Geometry: final body of the model. Coordinates: model frame, mm. Face numbers are marked on the shaded views. A direction names the side the tool comes from. Coordinates: 2 decimals unless noted, no trailing zeros. Loops run counter-clockwise (first coordinate to the right, second up) from the corner with the lowest first, then second, coordinate; pieces in that order, holes last. Notation, with made-up numbers: (75.5, 4) - (92.5, 4) arc R27 cw to (92.5, 27) - close; hole circle Ø10 at (60.25, 49.5). An arc over 180 degrees is marked (long way). Return JSON: item names as keys, results as strings.
from build123d import *

# Parameters (mm, degrees)
F0_W      = 822.325
F0_H      = 177.8
F1_DEPTH  = 228.6
F2_T      = -19.05
F3_W      = 784.225
F3_H      = 209.55
F4_DEPTH  = 6.35
F5_W      = 158.75
F5_H      = 209.55
F6_DEPTH  = 6.35
F7_W      = 158.75
F7_H      = 209.55
F8_DEPTH  = 6.35
F9_W      = 784.225
F9_H      = 158.75
F10_DEPTH = 6.35


with BuildPart() as f1:
    # F0 (on Top) → F1 (new body)
    with BuildSketch(Plane.XY):
        Rectangle(F0_W, F0_H)
    extrude(amount=F1_DEPTH)

    # F2
    f2_openings = [f1.faces().sort_by_distance(p)[0] for p in [
        (0, 0, 0),
    ]]
    offset(amount=F2_T, openings=f2_openings)

    # F3 (on face) → F4 (cut)
    with BuildSketch(Plane.XZ.offset(88.9)):
        with Locations((0.143385, 104.775)):
            Rectangle(F3_W, F3_H)
    extrude(amount=-F4_DEPTH, mode=Mode.SUBTRACT)

    # F5 (on face) → F6 (cut)
    with BuildSketch(Plane(origin=(-411.1625, 0, 0), x_dir=(0, -1, 0), z_dir=(-1, 0, 0))):
        with Locations((-9.525, 104.775)):
            Rectangle(F5_W, F5_H)
    extrude(amount=-F6_DEPTH, mode=Mode.SUBTRACT)

    # F7 (on face) → F8 (cut)
    with BuildSketch(Plane.YZ.offset(411.1625)):
        with Locations((9.525, 104.775)):
            Rectangle(F7_W, F7_H)
    extrude(amount=-F8_DEPTH, mode=Mode.SUBTRACT)

    # F9 (on face) → F10 (cut)
    with BuildSketch(Plane.XY.offset(228.6)):
        with Locations((0, 9.525)):
            Rectangle(F9_W, F9_H)
    extrude(amount=-F10_DEPTH, mode=Mode.SUBTRACT)


solid = f1.part
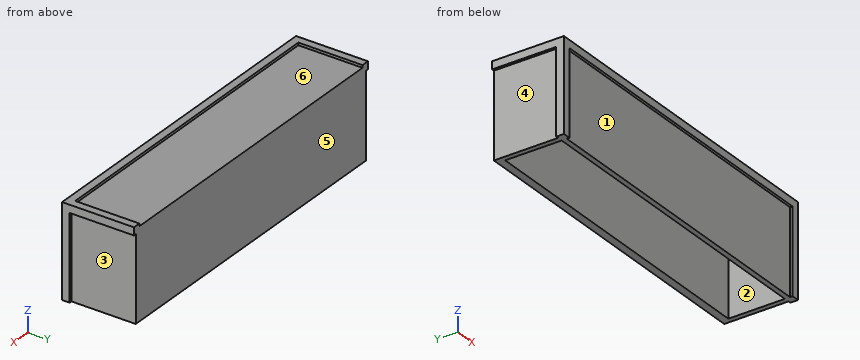
Item 1: First-contact query: pin 1 Ø3 at (y, z) = (50.5, 191.5) entering from -X; pin 2 Ø1.9 at (x, z) = (409, 112.5) entering from +Y; pin 3 Ø1.9 at (x, y) = (67, -87.5) entering from -Z. Flat tips, straight axial feed; report the tip coordinate or a pass-through.
Worked out:
{"pin 1": "x = -404.81", "pin 2": "y = -69.85", "pin 3": "z = 209.55"}
Item 2: Reachability of the marked faces 1, 2 and 3 from +Z, -Z, +X, -X, +Y, -Y: full face, straight path, thin tool, end or side. Return the list, or none.
Worked out:
{"face 1": "-Z, -Y", "face 2": "-Z", "face 3": "-Z, +X, +Y"}
Item 3: Ray query, probe 1 along X at (y, z) = (54, 103); probe 2 along Y at (x, z) = (-187, 156); probe 3 along Z at (x, y) = (194.5, 71). Return the intervals inside material, ascending. Write a range as from..to.
Worked out:
{"probe 1": "-404.81..-392.11, 392.11..404.81", "probe 2": "-82.55..-69.85, 69.85..88.9", "probe 3": "0..222.25"}
Item 4: Section query C-C, the plane x = 104.5. Return loops of the section in (y, z), and give its area (3 significant figures).
Worked out:
{"outline": "(-88.9, 209.55) - (-82.55, 209.55) - (-82.55, 0) - (-69.85, 0) - (-69.85, 209.55) - (69.85, 209.55) - (69.85, 0) - (88.9, 0) - (88.9, 222.25) - (-69.85, 222.25) - (-69.85, 228.6) - (-88.9, 228.6) - close", "area": "9,030 mm^2"}
Item 5: Mould query, pull axis X, two halves, no side actions, for the marked faces 4, 5 and 6. Classes: +X half, -X half, draft (parallel to the pull), parting line (faces both ways), or undercut.
Worked out:
{"face 4": "-X half", "face 5": "draft", "face 6": "undercut"}
Item 6: Section query A-A, the plane z = 195.5. Return loops of the section in (x, y).
Worked out:
{"outline": "(-411.16, -88.9) - (-391.97, -88.9) - (-391.97, -82.55) - (392.26, -82.55) - (392.26, -88.9) - (411.16, -88.9) - (411.16, -69.85) - (404.81, -69.85) - (404.81, 88.9) - (-404.81, 88.9) - (-404.81, -69.85) - (-411.16, -69.85) - close; hole (-392.11, -69.85) - (392.11, -69.85) - (392.11, 69.85) - (-392.11, 69.85) - close"}
Item 7: Section query B-B, the plane y = 52.5. Return loops of the section in (x, z), and give its area (3 significant figures).
Worked out:
{"outline": "(-411.16, 209.55) - (-404.81, 209.55) - (-404.81, 0) - (-392.11, 0) - (-392.11, 209.55) - (392.11, 209.55) - (392.11, 0) - (404.81, 0) - (404.81, 209.55) - (411.16, 209.55) - (411.16, 228.6) - (392.11, 228.6) - (392.11, 222.25) - (-392.11, 222.25) - (-392.11, 228.6) - (-411.16, 228.6) - close", "area": "16,000 mm^2"}
